The drawing under review shows one solid part. Ordinate dimensions are in mm from its lowest x, y, z. Give positions to 0.01 mm unless a question says otherwise; leave off trailing zeros. Loops run counter-clockwise (first coordinate to the right, second up) from the corner with the lowest first, then second, coordinate; pieces in that order, holes last. Notation, with made-up numbers: (-21.75, 68.25) - (-15.75, 68.25) arc R29 cw to (-15.75, 100.25) - close; hole circle Ø9 at (-33, -11). An arc over 180 degrees is marked (long way). Answer as CSV lines item,"result".
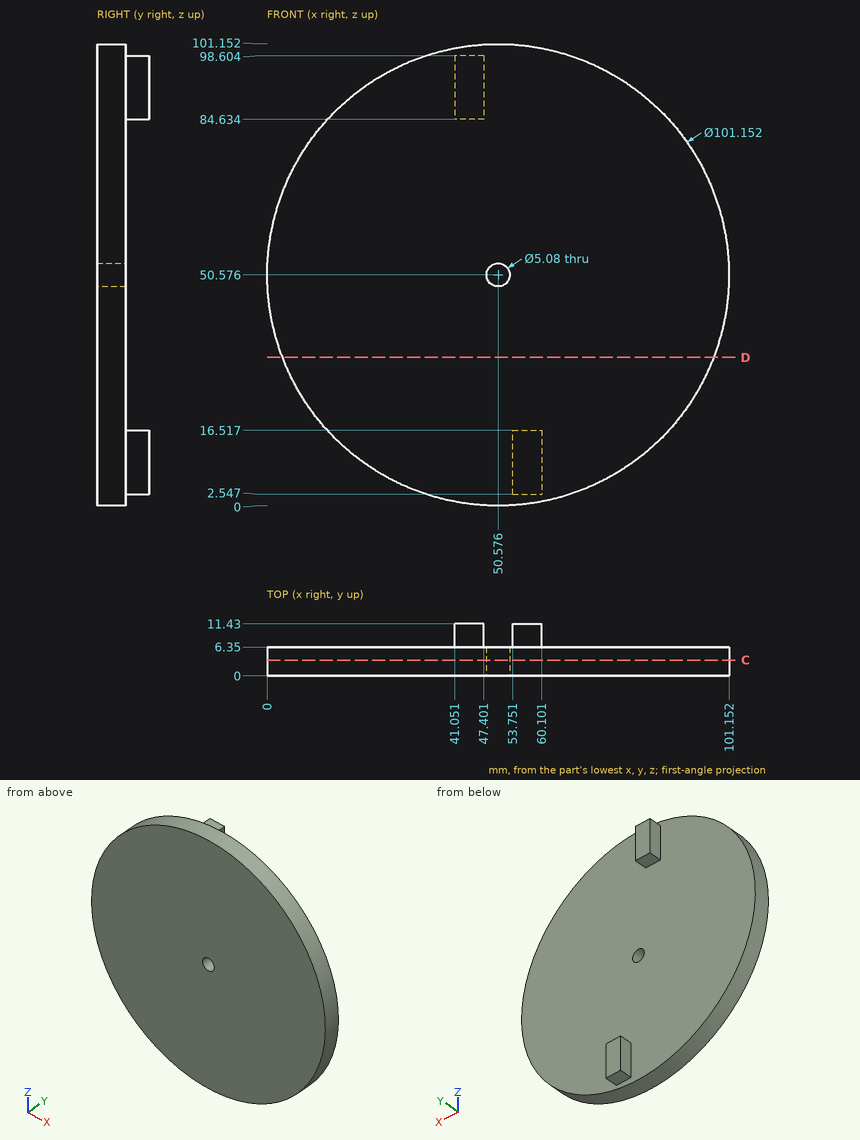
1) Insertion check: P1, Ø4, axis at y = 4.5, z = 24, coming from the +X side; P2, Ø5.5, axis at x = 45, y = 8.5, coming from the -Z side; P3, Ø5.5, axis at y = 8.5, z = 13, coming from the -X side. Each pin has a flat end and moves straight along its axis. Give the tip position at first contact, or say it passes through.
From the geometry:
P1,"stops at x = 94.78"
P2,"stops at z = 0.15"
P3,"stops at x = 14.91"
2) Consider section D-D on z = 32.5. Write out the cut boundary in (x, y).
From the geometry:
outline,"(3.34, 0) - (97.81, 0) - (97.81, 6.35) - (3.34, 6.35) - close"
3) Wall thickness on line 1 (Y direction, x = 91.5, z = 55.5); line 2 (X direction, y = 7.5, z = 91.5); line 3 (X direction, y = 10.25, z = 9): over which ranges is each line inside the solid? List them lowest first. Write a range as from..to.
From the geometry:
line 1,"y = 0..6.35"
line 2,"x = 41.05..47.4"
line 3,"x = 53.75..60.1"
4) Consider section C-C on y = 3.5. Write out the cut boundary in (x, z) (1 decimal), and give its area (3 significant figures).
From the geometry:
outline,"circle Ø101.2 at (50.6, 50.6); hole circle Ø5.1 at (50.6, 50.6)"
area,"8,020 mm^2"
